Check sheet for the modelled part. Datum: model origin and axes. Units: mm. Face numbers are marked on the shaded views. Round coordinates to 2 decimals unless told otherwise and drop trailing zeros. Order: outer loops, then holes, each group sorted by start corner. A loop starts at its lowest first (then second) coordinate and runs counter-clockwise, first axis right, second up.
Q1. Cross-section at A-A on z = 0. Record the cut outline in (x, y).
Q2. Cross-section at B-B on y = 0. Record the cut outline in (x, z) (3 decimals).
Q3. Cross-section at D-D on x = 115.5. Record the cut outline in (y, z).
Q4. Cross-section at C-C on x = 95.5. Record the cut outline in (y, z), then the cut area to 3 significant figures.
Q5. Scan lines: probe 1 along X at (y, z) = (-1, 0); probe 2 along Z at (x, y) = (14, 0) (3 decimals); probe 3 along X at (y, z) = (11, 0). Record each from-to range of solid material in increasing order.
Q6. Depth check by flat-ended pin: P1, Ø2.5, axis at y = -0.5, z = -0.5, coming from the -X side; P2, Ø3, axis at y = -9.5, z = 1, coming from the -X side; P3, Ø6, axis at x = 82, y = 12.5, coming from the +Z side. Enter the tip coordinate at first touch or a pass-through.
Q7. Mould release check, pull along X, two halves, no side actions. Record for the marked faces 1, 2 and 3: +X half, -X half, draft (parallel to the pull), parting line (faces both ways), or undercut.
from build123d import *

# Parameters (mm, degrees)
F1_DEPTH = 76.2
F2_R     = 25.4
F3_DEPTH = 76.2
F4_R     = 2.65
F5_DEPTH = 25.4
F6_R     = 12.7
F7_DEPTH = 25.4
F8_SIZE  = 5.08


with BuildPart() as f1:
    # F0 (on Right) → F1 (new body)
    with BuildSketch(Plane.YZ):
        with BuildLine():
            Line((-3.175, 3.175), (-3.175, 5.499261314))
            ThreePointArc((-3.175, 5.499261314), (0, -6.35), (3.175, 5.499261314))
            Line((3.175, 5.499261314), (3.175, 3.175))
            Line((3.175, 3.175), (-3.175, 3.175))
        make_face()
    extrude(amount=F1_DEPTH)

    # F2 (on face) → F3 (join)
    with BuildSketch(Plane.YZ.offset(76.2)):
        Circle(F2_R)
    extrude(amount=F3_DEPTH)

    # F4 (on face) → F5 (cut)
    with BuildSketch(Plane(origin=(0, 0, 0), x_dir=(0, -1, 0), z_dir=(-1, 0, 0))):
        Circle(F4_R)
    extrude(amount=-F5_DEPTH, mode=Mode.SUBTRACT)

    # F6 (on Front) → F7 (cut, symmetric)
    with BuildSketch(Plane.XZ):
        with Locations((121.220822216, 0)):
            Circle(F6_R)
    extrude(amount=F7_DEPTH, both=True, mode=Mode.SUBTRACT)

    # F8
    f8_edges = [f1.edges().sort_by_distance(p)[0] for p in [
        (152.4, -25.4, 0),
    ]]
    chamfer(f8_edges, length=F8_SIZE)


solid = f1.part
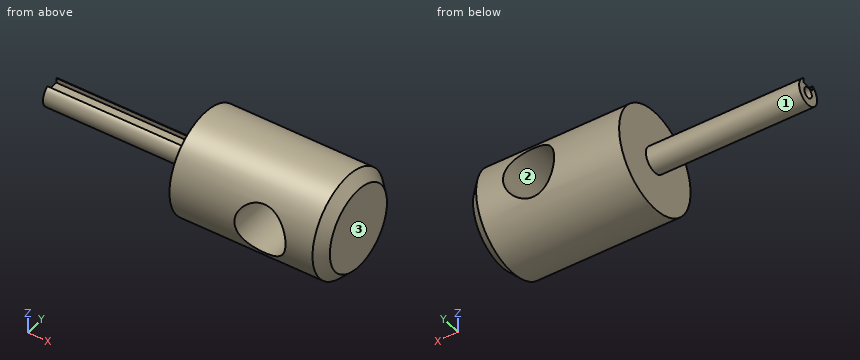
Results found:
1. outline: (0, -6.35) - (76.2, -6.35) - (76.2, -25.4) - (108.52, -25.4) - (108.52, 25.4) - (76.2, 25.4) - (76.2, 6.35) - (0, 6.35) - (0, 2.65) - (25.4, 2.65) - (25.4, -2.65) - (0, -2.65) - close; (133.92, -25.4) - (147.32, -25.4) - (152.4, -20.32) - (152.4, 20.32) - (147.32, 25.4) - (133.92, 25.4) - close
2. outline: (0, -6.35) - (76.2, -6.35) - (76.2, -25.4) - (147.32, -25.4) - (152.4, -20.32) - (152.4, 20.32) - (147.32, 25.4) - (76.2, 25.4) - (76.2, 3.175) - (0, 3.175) - (0, 2.65) - (25.4, 2.65) - (25.4, -2.65) - (0, -2.65) - close; hole circle Ø25.4 at (121.221, 0)
3. outline: (-22.73, -11.34) arc R25.4 ccw to (22.73, -11.34) - close; (-22.73, 11.34) - (22.73, 11.34) arc R25.4 ccw to start
4. outline: circle Ø50.8 at (0, 0)
4. area: 2,030 mm2
5. probe 1: x = 25.4 to 108.52, 133.92 to 152.4
5. probe 2: z = -6.35 to -2.65, 2.65 to 3.175
5. probe 3: x = 76.2 to 108.52, 133.92 to 152.4
6. P1: stops at x = 25.4
6. P2: stops at x = 76.2
6. P3: stops at z = 23.56
7. face 1: draft
7. face 2: undercut
7. face 3: +X half
